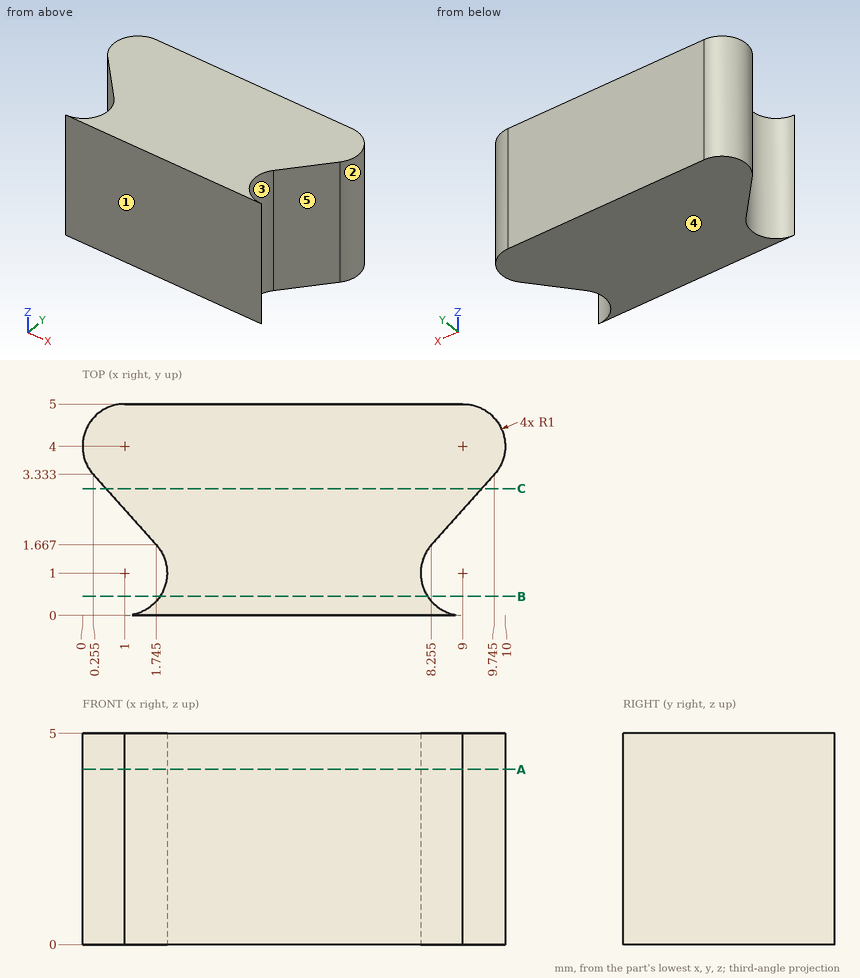
The drawing under review shows one solid part. Ordinate dimensions are in mm from its lowest x, y, z. A direction names the side the tool comes from. Coordinates: 2 decimals unless noted, no trailing zeros. Write each loop counter-clockwise with the first axis right and the second up, starting at its lowest first coordinate (ties: lowest second). Pieces come first, ordered by that corner, then holes. Notation, with made-up numbers: (61.25, 5) - (65.25, 5) arc R27 cw to (65.25, 41) - close; hole circle Ø3 at (26, 53.5). An arc over 180 degrees is marked (long way). Put each result on its own line as item: value.
1. Mouldability with a two-part tool opening along Y and no side actions: class the marked faces 1, 2 and 3 as released by +Y, released by -Y, zero draft, split by the parting line, or undercut.
Values found:
face 1: released by -Y
face 2: split by the parting line
face 3: undercut
2. Add section A-A, the plane z = 4.15. Give the boundary of the cut face in (x, y) (1 decimal).
Values found:
outline: (0.3, 3.3) - (1.7, 1.7) arc R1 cw to (1, 0) - (9, 0) arc R1 cw to (8.3, 1.7) - (9.7, 3.3) arc R1 ccw to (9, 5) - (1, 5) arc R1 ccw to start
3. Add section C-C, the plane y = 3. Give the boundary of the cut face in (x, z), then the cut area to 3 significant figures.
Values found:
outline: (0.55, 0) - (9.45, 0) - (9.45, 5) - (0.55, 5) - close
area: 44.5 mm²
4. Wall thickness on probe 1 along X at (y, z) = (2.5, 1.7); probe 2 along X at (y, z) = (0.85, 0.3); probe 3 along Y at (x, z) = (1.75, 2.65): over which ranges is each line inside the solid? List them lowest first.
Values found:
probe 1: 1 to 9
probe 2: 1.99 to 8.01
probe 3: 0 to 0.34, 1.66 to 5
5. Machinability: for the marked faces 4 and 5, which of the approach directions +Z, -Z, +X, -X, +Y, -Y give a long, thin tool a straight path to every point of the face, cutting with its end or side? Answer none if there is none.
Values found:
face 4: -Z, +X, -X, +Y, -Y
face 5: +Z, -Z, +X
6. Add section B-B, the plane y = 0.45. Give the boundary of the cut face in (x, z) (1 decimal).
Values found:
outline: (1.8, 0) - (8.2, 0) - (8.2, 5) - (1.8, 5) - close
